Model file for the job. Use its own axes, mm. A direction names the side the tool comes from. Give positions to 0.01 mm unless a question says otherwise; leave off trailing zeros. Write each loop counter-clockwise with the first axis right and the second up, starting at its lowest first coordinate (ties: lowest second). Pieces come first, ordered by that corner, then holes. Notation, with made-up numbers: (23, 23.25) - (42, 23.25) arc R32 ccw to (42, 58.25) - close; hole circle Ø5 at (-21.5, 6). An arc over 180 degrees is marked (long way). One line per item, written item: value. Start each with the question number.
(1) Cut at A-A, the plane x = 0. List the corners of the cut face in (y, z).
(2) Drop flat-ended pins along their axis: P1, Ø4, axis at y = 17, z = -23.5, coming from the -X side; P2, Ø5, axis at x = 0.5, z = 5.5, coming from the +Y side; P3, Ø5, axis at x = 13, y = 16.5, coming from the +Z side. Give the stop position or say it passes through.
(3) Probe L1, parallel to Z at x = 0, y = 3; L2, parallel to Y at x = 26, z = -6; L3, parallel to Z at x = 10.5, y = 16.25. List the from-to ranges inside material, lowest first.
(4) Cut at B-B, the plane z = 0. List the corners of the cut face in (x, y).
(5) Cut at C-C, the plane y = 15. List the corners of the cut face in (x, z).
(6) 3-axis set-ups, long thin cutter, end or side, ignore diameter. For faces 1 (the face through (16, 15, -20)), 2 (the face through (2.5, 15, -23)), 3 (the face through (16, 20, -23)): which of +Z, -Z, +X, -X, +Y, -Y reach the whole face in a straight line?
(7) Cut at D-D, the plane x = 7. List the corners of the cut face in (y, z), and give its area (3 significant figures).
(8) Mould opens along X. For faces 4 (the face through (0, 5, 1)), 5 (the face through (-30, 5, 0)), 6 (the face through (0, 5, 25)), 7 (the face through (30, 5, 0)) say: pulls with the +X half, pulls with the -X half, needs draft (parallel to the pull), parting line crosses it, or undercut.
from build123d import *

# Parameters (mm, degrees)
SKETCH1_W             = 60
SKETCH1_H             = 50
BOSS_EXTRUDE1_DEPTH   = 20
CUT_EXTRUDE1_DEPTH    = 10
F_2MM_DIAMETER_HOLE_D = 2


with BuildPart() as part:
    # Sketch1 → Boss-Extrude1 (new body)
    with BuildSketch(Plane(origin=(0, 0, 0), x_dir=(1, 0, 0), z_dir=(0, 1, 0))):
        Rectangle(SKETCH1_W, SKETCH1_H)
    extrude(amount=BOSS_EXTRUDE1_DEPTH)

    # Sketch2 → Cut-Extrude1 (cut)
    with BuildSketch(Plane(origin=(0, 20, 0), x_dir=(1, 0, 0), z_dir=(0, 1, 0))):
        Polygon((-30, 25), (2.5, 25), (2.5, 20), (30, 20), (30, -25), (2.5, -25), (-30, -25), align=None)
    extrude(amount=-CUT_EXTRUDE1_DEPTH, mode=Mode.SUBTRACT)

    # 2mm Diameter Hole (through all)
    with Locations(Plane(origin=(0, 10, 0), x_dir=(1, 0, 0), z_dir=(0, 1, 0))):
        with Locations((0, 0)):
            Hole(F_2MM_DIAMETER_HOLE_D / 2)


solid = part.part
Answers follow:
1. outline: (0, -25) - (10, -25) - (10, -1) - (0, -1) - close; (0, 1) - (10, 1) - (10, 25) - (0, 25) - close
2. P1: stops at x = 2.5
2. P2: stops at y = 10
2. P3: stops at z = -20
3. L1: z = -25 to -1, 1 to 25
3. L2: y = 0 to 10
3. L3: z = -25 to -20
4. outline: (-30, 0) - (-1, 0) - (-1, 10) - (-30, 10) - close; (1, 0) - (30, 0) - (30, 10) - (1, 10) - close
5. outline: (2.5, -25) - (30, -25) - (30, -20) - (2.5, -20) - close
6. face 1: +Z, +X, -X, +Y
6. face 2: +Z, -Z, -X, +Y
6. face 3: +Z, -Z, +X, -X, +Y
7. outline: (0, -25) - (20, -25) - (20, -20) - (10, -20) - (10, 25) - (0, 25) - close
7. area: 550 mm²
8. face 4: undercut
8. face 5: pulls with the -X half
8. face 6: needs draft
8. face 7: pulls with the +X half
